Autodesk Inventor part; units mm, degrees
ref_plane "YZ Plane" through (0, 0, 0) normal (1, 0, 0) x (0, 1, 0)
ref_plane "XZ Plane" through (0, 0, 0) normal (0, 1, 0) x (-1, 0, 0)
ref_plane "XY Plane" through (0, 0, 0) normal (0, 0, 1) x (1, 0, 0)
sketch "Sketch1" plane through (0, 0, 0) normal (0, 0, 1) x (1, 0, 0)
  circle A0 centre (0, 0) radius 30
  dimension "d0" = 60
extrude "Extrusion1" add sketch "Sketch1" along normal blind 10
sketch "Sketch2" plane through (0, 0, 10) normal (0, 0, 1) x (1, 0, 0)
  circle A0 centre (0, 19.9929) radius 7.5
  circle A1 centre (0, 19.9929) radius 2.75
  point P0 (0, 0)
  dimension "d3" = 15
  dimension "d4" = 5.5
extrude "Extrusion2" add sketch "Sketch2" along normal blind 12
properties part number "Disc"
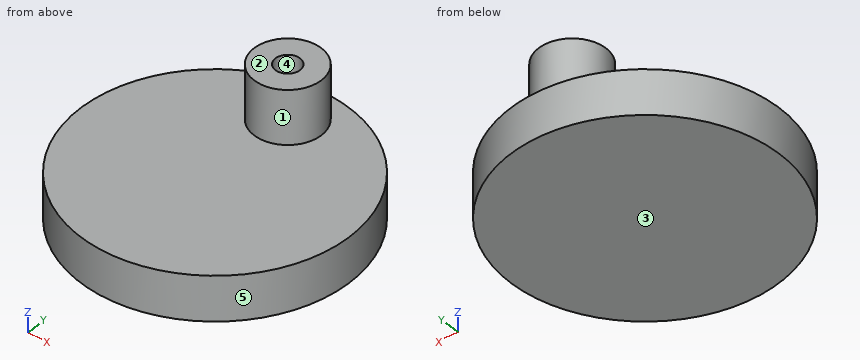
The listing builds one solid part. Answer for the finished solid, in the listing's coordinates (mm). Face numbers are marked on the shaded views. A direction names the side the tool comes from. Give positions to 0.01 mm unless a question says otherwise; leave off trailing zeros. Order: outer loops, then holes, each group sorted by start corner. A loop starts at its lowest first (then second) coordinate and runs counter-clockwise, first axis right, second up. Notation, with made-up numbers: (44, 37) - (89, 37) arc R24 cw to (89, 47) - close; hole circle Ø4 at (31, -6.5). An arc over 180 degrees is marked (long way). One line per item, written item: value. Start each with the question number.
1) A cutting plane is placed at B-B on y = 25. Give the vertices of the cut face in (x, z).
2) The mould has two halves that part along Y. Classify the marked faces 3, 4 and 5: released by +Y, released by -Y, zero draft, split by the parting line, or undercut.
3) A cutting plane is placed at A-A on x = 0. Give the vertices of the cut face in (y, z), then the cut area to 3 significant figures.
4) Given pin 1 Ø12 at (y, z) = (11.5, 11) entering from -X; pin 2 Ø18 at (x, y) = (-0.5, -7) entering from +Z; pin 3 Ø3 at (x, z) = (-6.5, 3) entering from +Y, each flat-ended and moving along its own axis, determine where each tip first touches the part or whether it passes through.
5) Find the intervals of material crossed by L1, parallel to Y at x = 0, z = 14; L2, parallel to Z at x = 6.5, y = -3; L3, parallel to X at y = 1, z = 8, in increasing order.
6) A cutting plane is placed at D-D on z = 11.25. Give the vertices of the cut face in (x, y), then the cut area to 3 significant figures.
7) A tool of negligible diameter and unlimited length cuts with its end or side. For the marked faces 1 and 2, from which of +Z, -Z, +X, -X, +Y, -Y can it reach the whole face along a straight path? Write none if from no direction.
8) A cutting plane is placed at C-C on z = 2. Give the vertices of the cut face in (x, y), then the cut area to 3 significant figures.
Answer sheet:
1. outline: (-16.58, 0) - (16.58, 0) - (16.58, 10) - (5.58, 10) - (5.58, 22) - (-5.58, 22) - (-5.58, 10) - (-16.58, 10) - close
2. face 3: zero draft
2. face 4: undercut
2. face 5: split by the parting line
3. outline: (-30, 0) - (30, 0) - (30, 10) - (27.49, 10) - (27.49, 22) - (22.74, 22) - (22.74, 10) - (17.24, 10) - (17.24, 22) - (12.49, 22) - (12.49, 10) - (-30, 10) - close
3. area: 714 mm2
4. pin 1: stops at x = -29.48
4. pin 2: stops at z = 10
4. pin 3: stops at y = 29.58
5. L1: y = 12.49 to 17.24, 22.74 to 27.49
5. L2: z = 0 to 10
5. L3: x = -29.98 to 29.98
6. outline: circle Ø15 at (0, 19.99); hole circle Ø5.5 at (0, 19.99)
6. area: 153 mm2
7. face 1: +Z
7. face 2: +Z, +X, -X, +Y, -Y
8. outline: circle Ø60 at (0, 0)
8. area: 2,830 mm2
